Solid Edge part; units mm, degrees
sketch "Sketch1" plane through (0, 0, 0) normal (0, 0, 1) x (1, 0, 0)
  line L0 (100, 0) -> (100, 50)
  line L1 (100, 50) -> (0, 50)
  line L2 (0, 50) -> (0, 0)
  line L3 (0, 0) -> (100, 0)
extrude "Protrusion1" add sketch "Sketch1" along normal blind 100
fillet "Round_1" radius 15 4 edges at (100, 25, 100) (0, 25, 100) (100, 25, 0) (0, 25, 0)
sketch "Sketch2" plane through (50, 0, 50) normal (0, -1, 0) x (1, 0, 0)
  line L0 (-35, 47.5) -> (35, 47.5)
  arc A0 (35, 47.5) -> (47.5, 35) centre (35, 35) cw
  line L1 (47.5, 35) -> (47.5, -35)
  arc A1 (47.5, -35) -> (35, -47.5) centre (35, -35) cw
  line L2 (35, -47.5) -> (-35, -47.5)
  arc A2 (-35, -47.5) -> (-47.5, -35) centre (-35, -35) cw
  line L3 (-47.5, -35) -> (-47.5, 35)
  arc A3 (-47.5, 35) -> (-35, 47.5) centre (-35, 35) cw
extrude "ExtrudedCutout_2" cut sketch "Sketch2" against normal blind 47.5
sketch "Sketch3" plane through (100, 25, 50) normal (1, 0, 0) x (0, 1, 0)
  line L0 (-25, 50) -> (-25, -50)
  line L1 (-25, -50) -> (-7.3673, 50)
  line L2 (-7.3673, 50) -> (-25, 50)
extrude "ExtrudedCutout_3" cut sketch "Sketch3" against normal blind 100
sketch "Sketch4" plane through (100, 26.3225, 50) normal (1, 0, 0) x (0, 1, 0)
  line L0 (23.6775, 0) -> (-26.3225, 0)
  line L1 (-26.3225, 0) -> (-26.3225, -50)
  line L2 (-26.3225, -50) -> (23.6775, -50)
  line L3 (23.6775, -50) -> (23.6775, 0)
extrude "ExtrudedCutout_4" cut sketch "Sketch4" against normal blind 108.373
fillet "Round_2" radius 1 5 edges at (100, 50, 67.5) (95.6066, 50, 95.6066) (50, 50, 100) (4.3934, 50, 95.6066) (0, 50, 67.5)
sketch "Sketch5" plane through (50, 13.2245, 75) normal (0, -0.9848, 0.1736) x (1, 0, 0)
  line L0 (-35.0001, 23.8471) -> (35, 23.8471)
  arc A0 (35, 23.8471) -> (48.5, 10.1545) centre (35, 10.3457) cw
  line L1 (48.5, 10.1545) -> (48.5, -25.3857)
  line L2 (-48.5, -25.3857) -> (48.5, -25.3857)
  line L3 (-48.5, -25.3857) -> (-48.5, 10.1543)
  arc A1 (-35.0001, 23.8471) -> (-48.5, 10.1543) centre (-35.0001, 10.3459) ccw
extrude "ExtrudedCutout_5" cut sketch "Sketch5" against normal blind 4
sketch "Sketch6" plane through (50, 13.2245, 75) normal (0, -0.9848, 0.1736) x (1, 0, 0)
  line L0 (47.5, 10.1618) -> (47.5, -24.3857)
  line L1 (47.5, -25.3857) -> (47.5, -24.3857)
  line L2 (48.5, -25.3857) -> (47.5, -25.3857)
  line L3 (48.5, 10.1545) -> (48.5, -25.3857)
  arc A0 (35, 23.8471) -> (48.5, 10.1545) centre (35, 10.3457) cw
  line L4 (-35.0001, 23.8471) -> (35, 23.8471)
  arc A1 (-35.0001, 23.8471) -> (-48.5, 10.1543) centre (-35.0001, 10.3459) ccw
  line L5 (-48.5, -25.3857) -> (-48.5, 10.1543)
  line L6 (-47.5, -25.3856) -> (-48.5, -25.3857)
  line L7 (-47.5, -24.3857) -> (-47.5, -25.3856)
  line L8 (-47.5, -24.3857) -> (-47.5, 10.1615)
  arc A2 (-47.5, 10.1615) -> (-35.0001, 22.8471) centre (-35.0001, 10.3459) cw
  line L9 (-35.0001, 22.8471) -> (35, 22.8471)
  arc A3 (35, 22.8471) -> (47.5, 10.1618) centre (35, 10.3457) cw
extrude "ExtrudedProtrusion_5" add sketch "Sketch6" against normal blind 1
sketch "Sketch7" plane through (50, 33.3163, 100) normal (0, 0, 1) x (0, 1, 0)
  line L0 (10.0492, -15) -> (10.0492, 15)
  line L1 (10.0492, 15) -> (0.0492, 15)
  line L2 (0.0492, 15) -> (0.0492, -15)
  line L3 (0.0492, -15) -> (10.0492, -15)
extrude "ExtrudedCutout_6" cut sketch "Sketch7" against normal blind 2.5
sketch "Sketch8" plane through (50, 33.6152, 97.5) normal (0, 0, -1) x (0, -1, 0)
  circle A0 centre (-4.7503, 18) radius 2.5
  circle A1 centre (-4.7503, -18) radius 2.5
extrude "ExtrudedProtrusion_6" add sketch "Sketch8" along normal blind 4
fillet "Round_3" radius 5 4 edges at (35, 33.3655, 98.75) (35, 43.3655, 98.75) (65, 33.3655, 98.75) (65, 43.3655, 98.75)
sketch "Sketch9" plane through (50, 32.3459, 97.5) normal (0, 0, -1) x (1, 0, 0)
  circle A0 centre (-32.5, -12.6508) radius 4.5
  circle A1 centre (-32.5, -12.6508) radius 1.5
  circle A2 centre (32.5, -12.6508) radius 4.5
  circle A3 centre (32.5, -12.6508) radius 1.5
extrude "ExtrudedProtrusion_7" add sketch "Sketch9" along normal blind 47.5
fillet "Round_4" radius 0.5 5 edges at (0, 11.9021, 67.5) (4.3934, 16.858, 95.6066) (50, 17.6327, 100) (95.6066, 16.858, 95.6066) (100, 11.9021, 67.5)
sketch "Sketch10" plane through (100, 29.162, 67.5) normal (1, 0, 0) x (0, 1, 0)
  line L0 (-5.958, -17.5) -> (-5.0897, -12.576)
  line L1 (-5.0897, -12.576) -> (-8.0442, -12.055)
  line L2 (-8.0442, -12.055) -> (-9.0042, -17.5)
  line L3 (-9.0042, -17.5) -> (-5.958, -17.5)
extrude "Cutout1" cut sketch "Sketch10" against normal blind 138.0733
sketch "Sketch11" plane through (100, 29.162, 67.5) normal (1, 0, 0) x (0, 1, 0)
  line L0 (-5.958, -17.5) -> (-5.0897, -12.576)
  line L1 (-5.0897, -12.576) -> (-8.0442, -12.055)
  line L2 (-8.0442, -12.055) -> (-9.0042, -17.5)
  line L3 (-9.0042, -17.5) -> (-5.958, -17.5)
extrude "ExtrudedProtrusion_8" add sketch "Sketch11" against normal blind 1.5
sketch "Sketch12" plane through (0, 29.162, 67.5) normal (-1, 0, 0) x (0, -1, 0)
  line L0 (5.0897, -12.576) -> (5.958, -17.5)
  line L1 (5.958, -17.5) -> (9.0042, -17.5)
  line L2 (9.0042, -17.5) -> (8.0442, -12.055)
  line L3 (8.0442, -12.055) -> (5.0897, -12.576)
extrude "ExtrudedProtrusion_9" add sketch "Sketch12" against normal blind 1.5
properties material "ABS Plastic, high impact"
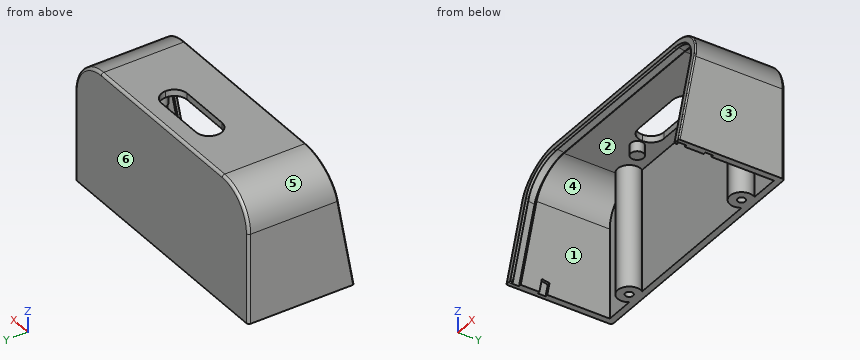
Check sheet for the modelled part. Datum: model origin and axes. Units: mm. Face numbers are marked on the shaded views. A direction names the side the tool comes from. Round coordinates to 2 decimals unless told otherwise and drop trailing zeros. Loops run counter-clockwise (first coordinate to the right, second up) from the corner with the lowest first, then second, coordinate; pieces in that order, holes last. Notation, with made-up numbers: M 40,69.5 L 98,69.5 A12 ccw 98,76.5 Z; hole C 26,36 d11. An arc over 180 degrees is marked long. One line per question, with ' | ' between items. Start each with the question number.
Item 1: Section check C-C (z = 53). State how many separate pieces and enclosed holes the cut face has, and give its area (3 significant figures).
Item 2: Section check B-B (x = 82.5). Record the boundary of the cut face in (y, z).
Item 3: Gauge pin test, flat ends, axial feed: pin 1 Ø0.9 at (x, y) = (82, 44.5) entering from -Z; pin 2 Ø2 at (y, z) = (19.5, 90.5) entering from +X; pin 3 Ø1.5 at (y, z) = (14.5, 92.5) entering from +X; pin 4 Ø4 at (x, y) = (67.5, 39) entering from -Z. Record the tip position at first contact, or that the pin passes through.
Item 4: Release check for a two-part mould opening along Y. For the marked faces 4, 5 and 6 record: released by +Y, released by -Y, zero draft, split by the parting line, or undercut.
Item 5: Set-up check for the marked faces 1, 2 and 3: record each of +Z, -Z, +X, -X, +Y, -Y from which the full face is reachable in a straight line by a thin tool's end or side.
Item 6: Section check D-D (x = 32). Record the boundary of the cut face in (y, z).
Item 7: Scan lines: probe 1 along Y at (x, z) = (82.5, 66.5); probe 2 along X at (y, z) = (29, 59.5); probe 3 along X at (y, z) = (41.5, 56). Record each from-to range of solid material in increasing order.
Item 8: Section check A-A (x = 57). Record the boundary of the cut face in (y, z), and give its area (3 significant figures).
Worked out:
1) separate pieces: 1 | enclosed holes: 2 | area: 520 mm^2
2) outline: M 17.19,97.5 L 18.18,97.33 L 18.35,98.31 L 21.3,97.79 L 21.25,97.5 L 40.5,97.5 L 40.5,50 L 43.5,50 L 43.5,97.5 L 46.5,97.5 L 46.5,50 L 50,50 L 50,99 A1 ccw 49,100 L 18.05,100 A0.5 ccw 17.56,99.59 Z
3) pin 1: z = 97.5 | pin 2: x = 99.31 | pin 3: through | pin 4: z = 93.5
4) face 4: undercut | face 5: zero draft | face 6: released by +Y
5) face 1: -Z, -Y | face 2: -Z | face 3: +Z, -Z, +X, +Y, -Y
6) outline: M 17.19,97.5 L 18.18,97.33 L 18.35,98.31 L 21.3,97.79 L 21.25,97.5 L 35.87,97.5 L 35.87,93.5 L 40.87,93.5 L 40.87,97.5 L 47.5,97.5 L 47.5,50 L 50,50 L 50,99 A1 ccw 49,100 L 18.05,100 A0.5 ccw 17.56,99.59 Z
7) probe 1: 40.5 to 43.5, 46.5 to 50 | probe 2: 0 to 2.5, 97.5 to 100 | probe 3: 0 to 2.5, 14.67 to 20.33, 79.67 to 85.33, 97.5 to 100
8) outline: M 17.19,97.5 L 18.18,97.33 L 18.35,98.31 L 21.3,97.79 L 21.25,97.5 L 33.37,97.5 L 33.37,100 L 18.05,100 A0.5 ccw 17.56,99.59 Z; M 43.37,97.5 L 47.5,97.5 L 47.5,50 L 50,50 L 50,99 A1 ccw 49,100 L 43.37,100 Z | area: 173 mm^2
